from build123d import *

# Parameters (mm, degrees)
SKETCH_2_R       = 50
EXTRUDE_1_DEPTH  = 3
SKETCH_3_R       = 27.5
EXTRUDE_2_DEPTH  = 1
SKETCH_4_R       = 15
EXTRUDE_3_DEPTH  = 1
SKETCH_5_R       = 7.5
EXTRUDE_4_DEPTH  = 1
EXTRUDE_5_DEPTH  = 3
SKETCH_16_W      = 15
SKETCH_16_H      = 5
EXTRUDE_7_DEPTH  = 20.52
SKETCH_18_W      = 15
SKETCH_18_H      = 5
EXTRUDE_9_DEPTH  = 20.55
SKETCH_19_W      = 33
SKETCH_19_H      = 5.022974077
EXTRUDE_10_DEPTH = 10
SKETCH_20_W      = 33
SKETCH_20_H      = 4.984152866
EXTRUDE_11_DEPTH = 10


with BuildPart() as part:
    # 草图2 → 凸台-拉伸1 (new body)
    with BuildSketch(Plane.XY):
        Circle(SKETCH_2_R)
    extrude(amount=EXTRUDE_1_DEPTH)

    # 草图3 → 凸台-拉伸2 (add)
    with BuildSketch(Plane.XY.offset(3)):
        Circle(SKETCH_3_R)
    extrude(amount=EXTRUDE_2_DEPTH)

    # 草图4 → 凸台-拉伸3 (add)
    with BuildSketch(Plane.XY.offset(4)):
        Circle(SKETCH_4_R)
    extrude(amount=EXTRUDE_3_DEPTH)

    # 草图5 → 凸台-拉伸4 (add)
    with BuildSketch(Plane.XY.offset(5)):
        Circle(SKETCH_5_R)
    extrude(amount=EXTRUDE_4_DEPTH)

    # 草图6 → 凸台-拉伸5 (add)
    with BuildSketch(Plane.XY):
        with BuildLine():
            Line((-12.491130148, -48.414581147), (-12.491130148, -114.964581147))
            Line((-12.491130148, -114.964581147), (8.028142932, -114.964581147))
            Line((8.028142932, -114.964581147), (8.028142932, -49.351280845))
            ThreePointArc((8.028142932, -49.351280845), (-2.280113003, -49.94798379), (-12.491130148, -48.414581147))
        make_face()
    extrude(amount=EXTRUDE_5_DEPTH)

    # 草图16 → 凸台-拉伸7 (add)
    with BuildSketch(Plane(origin=(8.028142932, 0, 0), x_dir=(0, 0, -1), z_dir=(1, 0, 0))):
        with Locations((7.5, -112.464581147)):
            Rectangle(SKETCH_16_W, SKETCH_16_H)
    extrude(amount=-EXTRUDE_7_DEPTH)

    # 草图18 → 凸台-拉伸9 (add)
    with BuildSketch(Plane(origin=(8.028142932, 0, 0), x_dir=(0, 0, -1), z_dir=(1, 0, 0))):
        with Locations((-10.5, -112.464581147)):
            Rectangle(SKETCH_18_W, SKETCH_18_H)
    extrude(amount=-EXTRUDE_9_DEPTH)

    # 草图19 → 凸台-拉伸10 (add)
    with BuildSketch(Plane(origin=(8.028142932, 0, 0), x_dir=(0, 0, -1), z_dir=(1, 0, 0))):
        with Locations((-1.5, -112.476068185)):
            Rectangle(SKETCH_19_W, SKETCH_19_H)
    extrude(amount=EXTRUDE_10_DEPTH)

    # 草图20 → 凸台-拉伸11 (add)
    with BuildSketch(Plane.ZY.offset(12.491857068)):
        with Locations((1.5, -112.45665758)):
            Rectangle(SKETCH_20_W, SKETCH_20_H)
    extrude(amount=EXTRUDE_11_DEPTH)


solid = part.part
Geometry check sheet. Reference: the model listing, model coordinates, mm. A direction names the side the tool comes from. Give positions to 0.01 mm unless a question says otherwise; leave off trailing zeros. Loops run counter-clockwise (first coordinate to the right, second up) from the corner with the lowest first, then second, coordinate; pieces in that order, holes last.
(1) Depth check by flat-ended pin: pin 1 Ø5.5 at (y, z) = (-112.5, 9) entering from +X; pin 2 Ø2.5 at (y, z) = (-92, 1) entering from +X; pin 3 Ø1 at (x, z) = (-32, -1.5) entering from -Y; pin 4 Ø6 at (x, z) = (-36, 5) entering from +Y. Enter the tip coordinate at first touch or a pass-through.
From the geometry:
pin 1: stops at x = 18.03
pin 2: stops at x = 8.03
pin 3: passes through
pin 4: stops at y = 36.88
(2) Set-up check for faces 1 (the flat face through (-1, -11, 0)), 2 (the flat face through (0, 0, 6)), 3 (the cylindrical face through (-5.961, -26.846, 3.493)): record each of +Z, -Z, +X, -X, +Y, -Y from which the full face is reachable in a straight line by a thin tool's end or side.
From the geometry:
face 1: -Z, +X, -X, +Y
face 2: +Z, +X, -X, +Y
face 3: +Z
(3) Section check C-C on y = 0. Record the cut outline in (x, z).
From the geometry:
outline: (-50, 0) - (50, 0) - (50, 3) - (27.5, 3) - (27.5, 4) - (15, 4) - (15, 5) - (7.5, 5) - (7.5, 6) - (-7.5, 6) - (-7.5, 5) - (-15, 5) - (-15, 4) - (-27.5, 4) - (-27.5, 3) - (-50, 3) - close
(4) Section check A-A on x = 0. Record the cut outline in (y, z).
From the geometry:
outline: (-114.96, -15) - (-109.96, -15) - (-109.96, 0) - (50, 0) - (50, 3) - (27.5, 3) - (27.5, 4) - (15, 4) - (15, 5) - (7.5, 5) - (7.5, 6) - (-7.5, 6) - (-7.5, 5) - (-15, 5) - (-15, 4) - (-27.5, 4) - (-27.5, 3) - (-109.96, 3) - (-109.96, 18) - (-114.96, 18) - close
(5) Thickness scan on L1, parallel to Y at x = -10, z = -5; L2, parallel to Z at x = 35, y = 7; L3, parallel to Z at x = 3, y = 14. Record the ranges inside material, lowest first.
From the geometry:
L1: y = -114.96 to -109.96
L2: z = 0 to 3
L3: z = 0 to 5
